```python
from build123d import *

# Parameters (mm, degrees)
SKETCH1_R           = 1.6
SKETCH1_W           = 119
SKETCH1_H           = 79
SKETCH1_W_2         = 21
SKETCH1_H_2         = 30
SKETCH1_W_3         = 3
SKETCH1_H_3         = 10
BOSS_EXTRUDE1_DEPTH = 3


with BuildPart() as part:
    # Sketch1 → Boss-Extrude1 (new body)
    with BuildSketch(Plane(origin=(0, 0, 0), x_dir=(1, 0, 0), z_dir=(0, 1, 0))):
        Polygon((0, 0), (194, 0), (194, 14.55), (194, 114.55), (194, 134), (0, 134), align=None)
        with Locations(Location((14, 103.5, 0), (0, 0, 270))):
            Circle(SKETCH1_R, mode=Mode.SUBTRACT)
        with Locations(Location((141, 103.5, 0), (0, 0, 270))):
            Circle(SKETCH1_R, mode=Mode.SUBTRACT)
        with Locations(Location((141, 25.5, 0), (0, 0, 270))):
            Circle(SKETCH1_R, mode=Mode.SUBTRACT)
        with Locations(Location((14, 25.5, 0), (0, 0, 270))):
            Circle(SKETCH1_R, mode=Mode.SUBTRACT)
        with Locations((77.5, 64.5)):
            Rectangle(SKETCH1_W, SKETCH1_H, mode=Mode.SUBTRACT)
        with Locations((156.5, 65)):
            Rectangle(SKETCH1_W_2, SKETCH1_H_2, mode=Mode.SUBTRACT)
        with Locations((4.5, 119)):
            Rectangle(SKETCH1_W_3, SKETCH1_H_3, mode=Mode.SUBTRACT)
        with Locations((4.5, 67)):
            Rectangle(SKETCH1_W_3, SKETCH1_H_3, mode=Mode.SUBTRACT)
        with Locations((4.5, 15)):
            Rectangle(SKETCH1_W_3, SKETCH1_H_3, mode=Mode.SUBTRACT)
        with Locations((189.5, 119)):
            Rectangle(SKETCH1_W_3, SKETCH1_H_3, mode=Mode.SUBTRACT)
        with Locations((189.5, 67)):
            Rectangle(SKETCH1_W_3, SKETCH1_H_3, mode=Mode.SUBTRACT)
        with Locations((189.5, 15)):
            Rectangle(SKETCH1_W_3, SKETCH1_H_3, mode=Mode.SUBTRACT)
    extrude(amount=BOSS_EXTRUDE1_DEPTH)


solid = part.part
```
Build history of the part. All positions in model axes, mm. Give positions to 0.01 mm unless a question says otherwise; leave off trailing zeros. Loops run counter-clockwise (first coordinate to the right, second up) from the corner with the lowest first, then second, coordinate; pieces in that order, holes last. Notation, with made-up numbers: (80.5, 65) -> (128.5, 65) arc R33 ccw to (128.5, 104) -> close; hole circle Ø5 at (19.5, 87). An arc over 180 degrees is marked (long way). One line per question, with ' | ' between items. Start each with the question number.
1) Cut at B-B (x = 92.5). Give the cut face in (y, z).
2) Cut at A-A (z = -95). Give the cut face in (x, y).
3) Cut at C-C (y = 1.8). Count the separate pieces of the cut face and the enclosed holes in it, plus the area to 3 significant figures.
4) Pin check, flat tip, straight feed: pin 1 (1 mm diameter, centred on x = 151, z = -43, fed in from -Y). Stop position of the tip, or through.
5) Probe L1, parallel to X at y = 0.25, z = -114.5; L2, parallel to Z at x = 141, y = 0.9; L3, parallel to X at y = 1.15, z = -55. List the from-to ranges inside material, lowest first.
Return value:
1) outline: (0, -134) -> (3, -134) -> (3, -104) -> (0, -104) -> close; (0, -25) -> (3, -25) -> (3, 0) -> (0, 0) -> close
2) outline: (0, 0) -> (18, 0) -> (18, 3) -> (0, 3) -> close; (137, 0) -> (194, 0) -> (194, 3) -> (137, 3) -> close
3) separate pieces: 1 | enclosed holes: 12 | area: 15,800 mm^2
4) pin 1: y = 0
5) L1: 0 to 3, 6 to 188, 191 to 194 | L2: -134 to -105.1, -101.9 to -27.1, -23.9 to 0 | L3: 0 to 18, 137 to 146, 167 to 194
